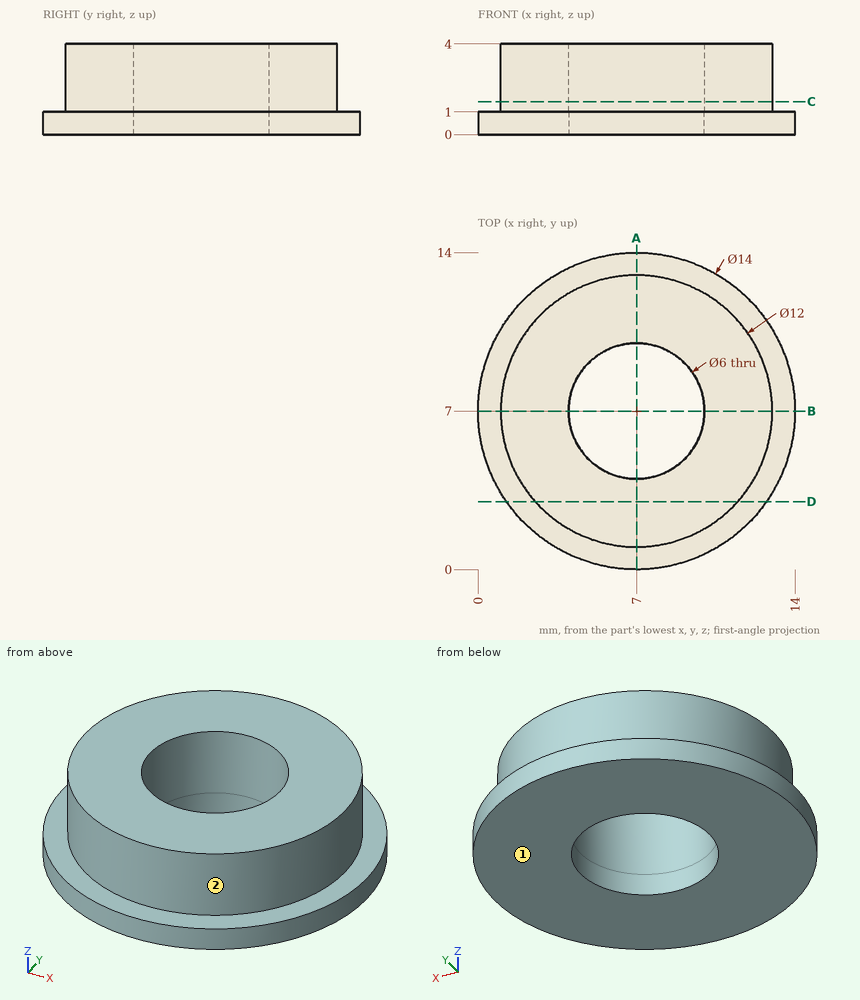
Check sheet for the drawn part. Datum: minimum x, y, z corner. Units: mm. A direction names the side the tool comes from. Coordinates: 2 decimals unless noted, no trailing zeros. Loops run counter-clockwise (first coordinate to the right, second up) from the corner with the lowest first, then second, coordinate; pieces in that order, holes last. Notation, with made-up numbers: (42, -25) -> (76, -25) arc R30 ccw to (76, 10) -> close; hole circle Ø9 at (68, 76.5). An arc over 180 degrees is marked (long way). Answer in a Markdown table with one row per item.
1) Section check D-D (y = 3). Record the cut outline in (x, z), and give its area (3 significant figures).
The answers:
| item | result |
|---|---|
| outline | (1.26, 0) -> (12.74, 0) -> (12.74, 1) -> (11.47, 1) -> (11.47, 4) -> (2.53, 4) -> (2.53, 1) -> (1.26, 1) -> close |
| area | 38.3 mm2 |
2) Scan lines: line 1 along Y through (x, z) = (7, 3.2); line 2 along Y through (x, z) = (7, 0.6); line 3 along Z through (x, y) = (12.5, 3.5). Record each from-to range of solid material in increasing order. Write a range as from..to.
The answers:
| item | result |
|---|---|
| line 1 | y = 1..4, 10..13 |
| line 2 | y = 0..4, 10..14 |
| line 3 | z = 0..1 |
3) Access from +Z, -Z, +X, -X, +Y, -Y to the whole of each face (thin tool, end or side, straight path). Record for the marked faces 1 and 2.
The answers:
| item | result |
|---|---|
| face 1 | -Z, +X, -X, +Y, -Y |
| face 2 | +Z |
4) Section check A-A (x = 7). Record the cut outline in (y, z).
The answers:
| item | result |
|---|---|
| outline | (0, 0) -> (4, 0) -> (4, 4) -> (1, 4) -> (1, 1) -> (0, 1) -> close; (10, 0) -> (14, 0) -> (14, 1) -> (13, 1) -> (13, 4) -> (10, 4) -> close |
5) Section check C-C (z = 1.45). Record the cut outline in (x, y).
The answers:
| item | result |
|---|---|
| outline | circle Ø12 at (7, 7); hole circle Ø6 at (7, 7) |
6) Depth check by flat-ended pin: P1, Ø1, axis at x = 9.5, z = 3.5, coming from the -Y side; P2, Ø1, axis at x = 3.5, z = 3, coming from the +Y side; P3, Ø2, axis at x = 9, z = 3, coming from the +Y side; P4, Ø1, axis at x = 7.5, y = 8, coming from the -Z side. Enter the tip coordinate at first touch or a pass-through.
The answers:
| item | result |
|---|---|
| P1 | stops at y = 1.34 |
| P2 | stops at y = 12.2 |
| P3 | stops at y = 12.92 |
| P4 | passes through |
